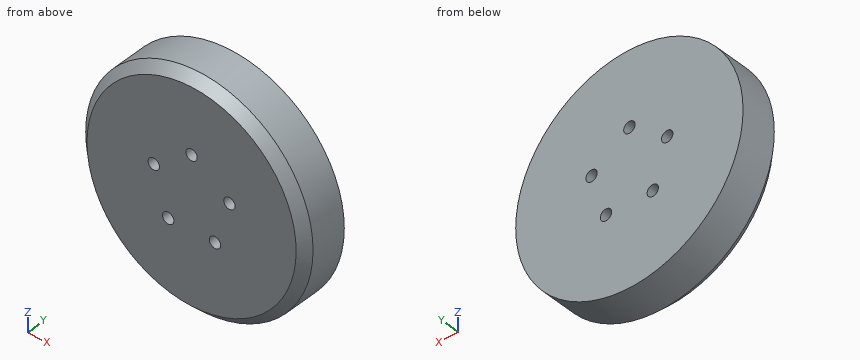
from build123d import *

# Parameters (mm, degrees)
F0_R     = 63.5
F1_DEPTH = 12.7
F3_D     = 6.35
F4_SIZE  = 5.08


with BuildPart() as f1:
    # F0 (on Front) → F1 (new body, symmetric)
    with BuildSketch(Plane.XZ):
        Circle(F0_R)
    extrude(amount=F1_DEPTH, both=True)

    # F3 (through all)
    with Locations(Plane.XZ.offset(12.7)):
        with Locations((0, 22.225), (21.137231, 6.867903), (13.063527, -17.980403), (-13.063527, -17.980403), (-21.137231, 6.867903)):
            Hole(F3_D / 2)

    # F4
    f4_edges = [f1.edges().sort_by_distance(p)[0] for p in [
        (-63.5, -12.7, 0),
    ]]
    chamfer(f4_edges, length=F4_SIZE)


solid = f1.part
Work out the finished part from the listing and answer in its coordinate system (mm). Give positions to 0.01 mm unless a question says otherwise; leave off trailing zeros. Loops run counter-clockwise (first coordinate to the right, second up) from the corner with the lowest first, then second, coordinate; pieces in that order, holes last. Notation, with made-up numbers: (44.25, -17.5) -> (58.25, -17.5) arc R25 ccw to (58.25, 5.5) -> close; hole circle Ø11 at (12.25, 74.5). An arc over 180 degrees is marked (long way). Use a Markdown table: item, result. Add a question column.
1) Each of these flat-tipped pins is pushed along its axis until it touches: P1, Ø6, axis at x = 13, y = 9, coming from the +Z side; P2, Ø12, axis at x = 41.5, y = 8, coming from the -Z side; P3, Ø3, axis at x = 40, y = -4.5, coming from the -Z side; P4, Ø4, axis at x = -13.06, z = -17.98, coming from the +Y side. Where does it stop, or does it pass through?
2) The part is cut by section C-C, the plane y = -9.25. Determine the outline of the cut face in (x, z) (3 decimals).
3) The part is cut by section B-B, the plane y = 11. Determine the outline of the cut face in (x, z) (3 decimals), plus the area to 3 significant figures.
4) The part is cut by section A-A, the plane x = 0. Determine the outline of the cut face in (y, z).
5) Consider line 1 along X through (y, z) = (11.75, -17.5); line 2 along X through (y, z) = (11.75, -15.5); line 3 along Z through (x, y) = (0, -1.25). Determine where each line is inside the solid, lowest interval first.
Reported:
| question | item | result |
|---|---|---|
| 1 | P1 | stops at z = 62.71 |
| 1 | P2 | stops at z = -52.65 |
| 1 | P3 | stops at z = -50.5 |
| 1 | P4 | passes through |
| 2 | outline | circle Ø123.74 at (0, 0); hole circle Ø6.35 at (-21.137, 6.868); hole circle Ø6.35 at (-13.064, -17.98); hole circle Ø6.35 at (0, 22.225); hole circle Ø6.35 at (13.064, -17.98); hole circle Ø6.35 at (21.137, 6.868) |
| 3 | outline | circle Ø127 at (0, 0); hole circle Ø6.35 at (-21.137, 6.868); hole circle Ø6.35 at (-13.064, -17.98); hole circle Ø6.35 at (0, 22.225); hole circle Ø6.35 at (13.064, -17.98); hole circle Ø6.35 at (21.137, 6.868) |
| 3 | area | 12,500 mm^2 |
| 4 | outline | (-12.7, -58.42) -> (-7.62, -63.5) -> (12.7, -63.5) -> (12.7, 19.05) -> (-12.7, 19.05) -> close; (-12.7, 25.4) -> (12.7, 25.4) -> (12.7, 63.5) -> (-7.62, 63.5) -> (-12.7, 58.42) -> close |
| 5 | line 1 | x = -61.04 to -16.2, -9.93 to 9.93, 16.2 to 61.04 |
| 5 | line 2 | x = -61.58 to -15.05, -11.08 to 11.08, 15.05 to 61.58 |
| 5 | line 3 | z = -63.5 to 19.05, 25.4 to 63.5 |
